Check sheet for the modelled part. Datum: model origin and axes. Units: mm. Face numbers are marked on the shaded views. A direction names the side the tool comes from. Round coordinates to 2 decimals unless told otherwise and drop trailing zeros. Loops run counter-clockwise (first coordinate to the right, second up) from the corner with the lowest first, then second, coordinate; pieces in that order, holes last. Notation, with made-up numbers: (63, 45) -> (114, 45) arc R18 cw to (114, 69) -> close; hole circle Ø9 at (40, 18). An arc over 180 degrees is marked (long way). Use one line per item in the form item = value. Start each with the question number.
(1) Material ranges on probe 1 along Z at (x, y) = (1.15, -14); probe 2 along Y at (x, z) = (2.8, -14.5); probe 3 along Y at (x, z) = (1.8, -3.5), recorded low to high. Write a range as [from, to].
(2) Sectioned sample at B-B (y = 0). Record the cut outline in (x, z), and give its area (3 significant figures).
(3) Sectioned sample at A-A (z = 0). Record the cut outline in (x, y).
(4) Draft check along Y on the marked faces 1, 2 and 3. Enter one of: released by +Y, released by -Y, zero draft, split by the parting line, or undercut.
(5) Go/stop test with a flat-tipped pin: pin 1 (1.5 mm diameter, centred on x = 1, y = 14, fed in from -Z). Record where the tip stops, or that it passes through.
(6) Set-up check for the marked faces 4, 5 and 6: record each of +Z, -Z, +X, -X, +Y, -Y from which the full face is reachable in a straight line by a thin tool's end or side.
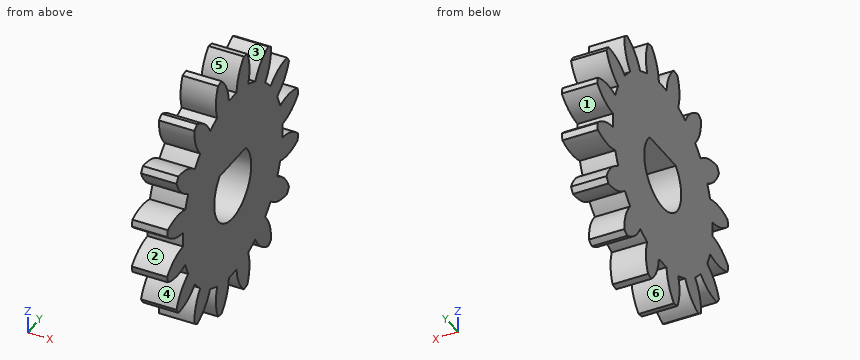
from build123d import *

# Parameters (mm, degrees)
BASPROSKE_W     = 5
BASPROSKE_H     = 18
TOOTHCUT_DEPTH  = 26.942243542
TEETHCUTS_COUNT = 16
TEETHCUTS_ANGLE = 337.5
BORSKE_R        = 5
BORE_DEPTH      = 50.0000508
EXTRUDE_START   = -5
EXTRUDE_1_DEPTH = 5


with BuildPart() as part:
    # BasProSke → Base-Revolve (revolve)
    with BuildSketch(Plane(origin=(0, 0, 0), x_dir=(1, 0, 0), z_dir=(0, 1, 0)), mode=Mode.PRIVATE) as base_revolve_sk:
        with Locations((2.5, 9)):
            Rectangle(BASPROSKE_W, BASPROSKE_H)
    revolve(base_revolve_sk.sketch.rotate(Axis((-10, 0, 0), (1, 0, 0)), 180), axis=Axis((-10, 0, 0), (1, 0, 0)))

    # TooCutSke → ToothCut (cut, through all)
    with BuildSketch(Plane(origin=(0, 0, 0), x_dir=(0, 0, -1), z_dir=(1, 0, 0))):
        with BuildLine():
            ThreePointArc((1.03434411, 13.459313997), (0, 13.499), (-1.03434411, 13.459313997))
            ThreePointArc((-1.03434411, 13.459313997), (-1.635143665, 15.806872195), (-3.065655864, 17.762792553))
            ThreePointArc((-3.065655864, 17.762792553), (0, 18.0254), (3.065655864, 17.762792553))
            ThreePointArc((3.065655864, 17.762792553), (1.635143665, 15.806872195), (1.03434411, 13.459313997))
        make_face()
    toothcut = extrude(amount=TOOTHCUT_DEPTH, mode=Mode.SUBTRACT)

    # TeethCuts: ToothCut ×16 about axis
    teethcuts_axis = Axis((-10, 0, 0), (1, 0, 0))
    for i in range(1, TEETHCUTS_COUNT):
        add(toothcut.rotate(teethcuts_axis, i * TEETHCUTS_ANGLE / (TEETHCUTS_COUNT - 1)), mode=Mode.SUBTRACT)

    # BorSke → Bore (cut, symmetric)
    with BuildSketch(Plane(origin=(0, 0, 0), x_dir=(0, 0, -1), z_dir=(1, 0, 0))):
        with Locations(Location((0, 0, 0), (0, 0, 180))):
            Circle(BORSKE_R)
    extrude(amount=BORE_DEPTH, both=True, mode=Mode.SUBTRACT)

    # 草图2 → 凸台-拉伸1 (add)
    with BuildSketch(Plane.ZY.offset(EXTRUDE_START)):
        with BuildLine():
            Line((3.544820497, 3.526222858), (3.544820497, -3.526222858))
            ThreePointArc((3.544820497, -3.526222858), (5, 0), (3.544820497, 3.526222858))
        make_face()
    extrude(amount=EXTRUDE_1_DEPTH)


solid = part.part
Checks:
q1.probe_1 = [-10.38, -7.58], [-4.48, -1.09], [1.09, 4.48], [7.58, 10.38]
q1.probe_2 = [-10.4, -8.22], [-4.53, -1.18], [1.18, 4.53], [8.22, 10.4]
q1.probe_3 = [-17.66, -3.57], [3.57, 17.66]
q2.outline = (0, -13.5) -> (5, -13.5) -> (5, -5) -> (0, -5) -> close; (0, 3.54) -> (5, 3.54) -> (5, 13.5) -> (0, 13.5) -> close
q2.area = 92.3 mm2
q3.outline = (0, -13.5) -> (5, -13.5) -> (5, -5) -> (0, -5) -> close; (0, 5) -> (5, 5) -> (5, 13.5) -> (0, 13.5) -> close
q4.face_1 = released by +Y
q4.face_2 = released by -Y
q4.face_3 = undercut
q5.pin_1 = -10.4
q6.face_4 = +X, -X, -Y
q6.face_5 = +Z, +X, -X
q6.face_6 = -Z, +X, -X
